Could you check a few things on this model? Use its own coordinates, in mm. A direction names the side the tool comes from. Give positions to 0.01 mm unless a question says otherwise; leave off trailing zeros. Write each loop counter-clockwise with the first axis right and the second up, starting at its lowest first coordinate (ties: lowest second). Pieces come first, ordered by that corner, then holes. Notation, with made-up numbers: (35.25, 29) - (45.25, 29) arc R10 cw to (45.25, 36) - close; hole circle Ø3 at (51, 60.25). An arc over 180 degrees is marked (long way). Use one line per item in the form item = value.
Autodesk Fusion 360 part; units mm, degrees
sketch "Sketch1" plane through (0, 0, 0) normal (0, 0, 1) x (1, 0, 0)
  line L0 (0, 0) -> (50, 0)
  line L1 (50, 0) -> (50, 50)
  line L2 (50, 50) -> (0, 50)
  line L3 (0, 50) -> (0, 0)
  circle A0 centre (8, 42) radius 2.25
  line L4 (8, 42) -> (42, 42) construction
  line L5 (42, 42) -> (42, 8) construction
  line L6 (42, 8) -> (8, 8) construction
  line L7 (8, 8) -> (8, 42) construction
  circle A1 centre (8, 8) radius 2.25
  circle A2 centre (42, 42) radius 2.25
  circle A3 centre (42, 8) radius 2.25
  circle A4 centre (25, 15) radius 5
  line L8 (25, 15) -> (25, 35) construction
  circle A5 centre (25, 35) radius 5
  circle A6 centre (25, 35) radius 2.5
  circle A7 centre (25, 20) radius 2.5
  line L9 (27.5, 15) -> (27.5, 35)
  line L10 (22.5, 15) -> (22.5, 35)
  line L11 (30, 15) -> (30, 35)
  line L12 (20, 15) -> (20, 35)
  dimension "d1" = 50
  dimension "d2" = 4.5
  dimension "d3" = 8
  dimension "d4" = 8
  dimension "d5" = 8
  dimension "d6" = 8
  dimension "d7" = 4.5
  dimension "d8" = 4.5
  dimension "d9" = 4.5
  dimension "d10" = 10
  dimension "d11" = 20
  dimension "d13" = 15
  dimension "d14" = 10
  dimension "d15" = 5
  dimension "d16" = 5
  dimension "d17" = 2.5
  dimension "d18" = -2.5
  dimension "d19" = 5
  dimension "d20" = -5
extrude "Extrude1" add sketch "Sketch1" along normal blind 7 contours L0 L1 L2 L3 | A4 A5 L10 L12 | A4 A5 L9 L11 | A5 A6 L9 L10 picked at (20.8519, 34.7516)
extrude "Extrude2" cut sketch "Sketch1" along normal blind 3.175 contours A4 A5 L10 L12 | A4 A5 L9 L11 | A5 A6 L9 L10 picked at (20.8519, 34.7516)
fillet "Fillet1" radius 3.175 4 edges at (0, 0, 3.5) (50, 0, 3.5) (50, 50, 3.5) (0, 50, 3.5)
chamfer "Chamfer1" distance 2 angle 45 4 edges at (5.9023, 42.8136, 7) (5.9023, 8.8136, 7) (39.9023, 8.8136, 7) (39.9023, 42.8136, 7)
sketch "Sketch2" plane through (0, 0, 3.175) normal (0, 0, -1) x (1, 0, 0)
  line L0 (22.5, -35) -> (22.5, -19.3301)
  arc A0 (20, -15) -> (22.5, -19.3301) centre (25, -15) ccw
  line L1 (20, -15) -> (20, -35)
  arc A1 (20, -35) -> (30, -35) centre (25, -35) ccw
  line L2 (30, -35) -> (30, -15)
  arc A2 (27.5, -19.3301) -> (30, -15) centre (25, -15) ccw
  line L3 (27.5, -19.3301) -> (27.5, -35)
  arc A3 (22.5, -35) -> (27.5, -35) centre (25, -35) ccw
  line L4 (20, -35) -> (20, -15)
  arc A4 (30, -15) -> (20, -15) centre (25, -15) ccw
  line L5 (30, -15) -> (30, -35)
  arc A5 (20, -35) -> (30, -35) centre (25, -35) ccw
1. Imagine slicing it at B-B, the plane x = 42. List the corners of the cut face in (y, z) for me.
Response values:
outline = (0, 0) - (5.75, 0) - (5.75, 5) - (3.75, 7) - (0, 7) - close; (10.25, 0) - (39.75, 0) - (39.75, 5) - (37.75, 7) - (12.25, 7) - (10.25, 5) - close; (44.25, 0) - (50, 0) - (50, 7) - (46.25, 7) - (44.25, 5) - close
2. If we mould it in two halves opening along X, with no side actions, what happens to faces 1 (the face through (49.05, 0.91, 3.55)), 2 (the face through (6.34, 6.48, 2.46)), 3 (the face through (0, 25, 3)), 4 (the face through (39.752, 7.901, 2.465))? For each: pulls with the +X half, pulls with the -X half, needs draft (parallel to the pull), parting line crosses it, or undercut.
Response values:
face_1 = pulls with the +X half
face_2 = undercut
face_3 = pulls with the -X half
face_4 = undercut
3. Imagine slicing it at A-A, the plane y = 23. List the corners of the cut face in (x, z) for me (3 decimals), and give its area (3 significant figures).
Response values:
outline = (0, 0) - (20, 0) - (20, 3.175) - (22.5, 3.175) - (22.5, 7) - (0, 7) - close; (27.5, 3.175) - (30, 3.175) - (30, 0) - (50, 0) - (50, 7) - (27.5, 7) - close
area = 299 mm²
4. If I drill on line 1 (Y direction, x = 42, z = 1.3); line 2 (X direction, y = 15, z = 5.75); line 3 (X direction, y = 19.5, z = 6.25), over which ranges is the centre line in solid material (lowest first)? Write a range as from..to.
Response values:
line_1 = 0..5.75, 10.25..39.75, 44.25..50
line_2 = 0..20, 30..50
line_3 = 0..22.5, 27.5..50
5. Which directions (+Z, -Z, +X, -X, +Y, -Y) give clear straight access to the entire face, cutting with the end or side of a thin tool? Please do faces 5 (the face through (24.9, 37.5, 5.1)), 6 (the face through (30, 25, 2)), 7 (the face through (19, 25, 0)).
Response values:
face_5 = +Z, -Z
face_6 = -Z
face_7 = -Z, +X, -X, +Y, -Y
6. For pin 1 (3 mm diameter, centred on x = 9, z = 1.5, fed in from -Y); pin 2 (3.5 mm diameter, centred on x = 8, y = 42, fed in from +Z); pin 3 (5 mm diameter, centred on x = 24.5, y = 26.5, fed in from -Z) (3 decimals), each with a flat end and sliding along its axis, tell me the tip position at first contact or that it passes through.
Response values:
pin_1 = 0
pin_2 = through
pin_3 = 3.175
7. Imagine slicing it at C-C, the plane z = 1. List the corners of the cut face in (x, y) for me (3 decimals), and give its area (3 significant figures).
Response values:
outline = (0, 3.175) arc R3.175 ccw to (3.175, 0) - (46.825, 0) arc R3.175 ccw to (50, 3.175) - (50, 46.825) arc R3.175 ccw to (46.825, 50) - (3.175, 50) arc R3.175 ccw to (0, 46.825) - close; hole circle Ø4.5 at (8, 8); hole circle Ø4.5 at (8, 42); hole (20, 15) arc R5 ccw to (30, 15) - (30, 35) arc R5 ccw to (20, 35) - close; hole circle Ø4.5 at (42, 8); hole circle Ø4.5 at (42, 42)
area = 2,150 mm²
